Build history of the part. All positions in model axes, mm. Round coordinates to 2 decimals unless told otherwise and drop trailing zeros. Loops run counter-clockwise (first coordinate to the right, second up) from the corner with the lowest first, then second, coordinate; pieces in that order, holes last. Notation, with made-up numbers: (45, 8.5) -> (80, 8.5) arc R25 ccw to (80, 31.5) -> close; hole circle Ø2 at (47.25, 45.5). An arc over 180 degrees is marked (long way). Put each result on its own line as item: value. Start each with the question number.
```python
from build123d import *

# Parameters (mm, degrees)
F1_DEPTH = 1450
F2_T     = -2
F4_D     = 6.5
F4_DEPTH = 25
F6_D     = 8
F8_D     = 8


with BuildPart() as f1:
    # F0 (on Top) → F1 (new body)
    with BuildSketch(Plane.XY):
        with BuildLine():
            ThreePointArc((-25, -22), (-24.12132, -24.12132), (-22, -25))
            Line((-22, -25), (22, -25))
            ThreePointArc((22, -25), (24.12132, -24.12132), (25, -22))
            Line((25, -22), (25, 22))
            ThreePointArc((25, 22), (24.12132, 24.12132), (22, 25))
            Line((22, 25), (-22, 25))
            ThreePointArc((-22, 25), (-24.12132, 24.12132), (-25, 22))
            Line((-25, 22), (-25, -22))
        make_face()
    extrude(amount=F1_DEPTH)

    # F2
    f2_openings = [f1.faces().sort_by_distance(p)[0] for p in [
        (0, 0, 1450),
        (0, 0, 0),
    ]]
    offset(amount=F2_T, openings=f2_openings)

    # F4
    with Locations(Plane.XZ.offset(25)):
        with Locations((0, 1420)):
            Hole(F4_D / 2, depth=F4_DEPTH)

    # F6 (through all)
    with Locations(Plane.XZ.offset(25)):
        with Locations((0, 60)):
            Hole(F6_D / 2)

    # F8 (through all)
    with Locations(Plane(origin=(-25, 0, 0), x_dir=(0, -1, 0), z_dir=(-1, 0, 0))):
        with Locations((0, 200)):
            Hole(F8_D / 2)


solid = f1.part
```
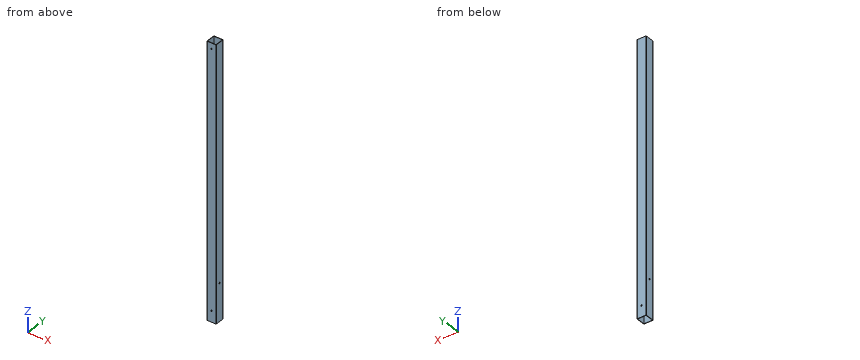
Item 1: Wall check: line 1 (Z direction, x = 0, y = -23.4); line 2 (X direction, y = 0.5, z = 1079.5). Give the ranges that are in metal, low to high. Write a range as from..to.
Item 2: Drop a flat-ended pin along its axis: pin 1 (8 mm diameter, centred on x = 16.5, y = -9.5, fed in from -Z). Give the stop position or say it passes through.
Item 3: Cut at A-A on y = 14. Write the cut outline in (x, z).
Item 4: Cut at B-B on z = 764. Write the cut outline in (x, y).
Ans:
1. line 1: z = 0..56, 64..1416.75, 1423.25..1450
1. line 2: x = -25..-23, 23..25
2. pin 1: passes through
3. outline: (-25, 0) -> (-23, 0) -> (-23, 1450) -> (-25, 1450) -> close; (23, 0) -> (25, 0) -> (25, 1450) -> (23, 1450) -> close
4. outline: (-25, -22) arc R3 ccw to (-22, -25) -> (22, -25) arc R3 ccw to (25, -22) -> (25, 22) arc R3 ccw to (22, 25) -> (-22, 25) arc R3 ccw to (-25, 22) -> close; hole (-23, -22) arc R1 ccw to (-22, -23) -> (22, -23) arc R1 ccw to (23, -22) -> (23, 22) arc R1 ccw to (22, 23) -> (-22, 23) arc R1 ccw to (-23, 22) -> close
